Read the model definition and answer for the solid it produces. Units are mm, in the model's axes. Face numbers are marked on the shaded views. A direction names the side the tool comes from. Give positions to 0.01 mm unless a question says otherwise; leave off trailing zeros. Loops run counter-clockwise (first coordinate to the right, second up) from the corner with the lowest first, then second, coordinate; pieces in that order, holes last. Notation, with made-up numbers: (-11.75, 22) -> (6.25, 22) arc R12 ccw to (6.25, 33) -> close; hole circle Ø8 at (-15.5, 27). An arc over 180 degrees is marked (long way). Return JSON: item names as keys, results as strings. Group by question number.
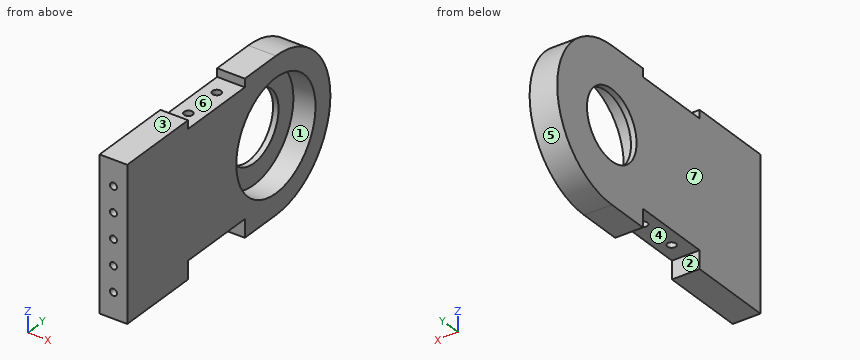
from build123d import *

# Parameters (mm, degrees)
BOSS_EXTRUDE1_DEPTH              = 20
SKETCH3_R                        = 40
CUT_EXTRUDE1_DEPTH               = 16
SKETCH4_R                        = 25
CUT_EXTRUDE2_DEPTH               = 11.1125
TAP_DRILL_FOR_M6X1_0_TAP2_D      = 5
TAP_DRILL_FOR_M6X1_0_TAP2_DEPTH  = 40
TAP_DRILL_FOR_M6X1_0_TAP2_TIP    = 1.502151548
SKETCH12_W                       = 6
SKETCH12_H                       = 57.3
SKETCH12_W_2                     = 13
CUT_EXTRUDE3_DEPTH               = 20
TAP_DRILL_FOR_M6_HELICOIL1_D     = 6.25
TAP_DRILL_FOR_M6_HELICOIL1_DEPTH = 20
TAP_DRILL_FOR_M6_HELICOIL1_TIP   = 1.877689434
TAP_DRILL_FOR_M6_HELICOIL2_D     = 6.25
TAP_DRILL_FOR_M6_HELICOIL2_DEPTH = 20
TAP_DRILL_FOR_M6_HELICOIL2_TIP   = 1.877689434


with BuildPart() as part:
    # Sketch2 → Boss-Extrude1 (new body)
    with BuildSketch(Plane(origin=(0, 0, 0), x_dir=(0, 0, -1), z_dir=(1, 0, 0))):
        with BuildLine():
            Line((55, -75), (55, 75))
            ThreePointArc((55, 75), (0, 20), (-55, 75))
            Line((-55, 75), (-55, -75))
            Line((-55, -75), (55, -75))
        make_face()
        with BuildLine():
            ThreePointArc((-55, 75), (0, 20), (55, 75))
            Line((55, 75), (-55, 75))
        make_face()
        with BuildLine():
            Line((-55, 75), (55, 75))
            ThreePointArc((55, 75), (0, 130), (-55, 75))
        make_face()
    extrude(amount=BOSS_EXTRUDE1_DEPTH)

    # Sketch3 → Cut-Extrude1 (cut)
    with BuildSketch(Plane(origin=(20, 0, 0), x_dir=(0, 0, -1), z_dir=(1, 0, 0))):
        with Locations((0, 75)):
            Circle(SKETCH3_R)
    extrude(amount=-CUT_EXTRUDE1_DEPTH, mode=Mode.SUBTRACT)

    # Sketch4 → Cut-Extrude2 (cut)
    with BuildSketch(Plane(origin=(4, 0, 0), x_dir=(0, 0, -1), z_dir=(1, 0, 0))):
        with Locations((0, 75)):
            Circle(SKETCH4_R)
    extrude(amount=-CUT_EXTRUDE2_DEPTH, mode=Mode.SUBTRACT)

    # Tap Drill for M6x1.0 Tap2
    with Locations(Plane(origin=(0, -75, 0), x_dir=(-1, 0, 0), z_dir=(0, -1, 0))):
        with Locations((-10, -36.666666667), (-10, -18.333333333), (-10, 0), (-10, 18.333333333), (-10, 36.666666667)):
            Hole(TAP_DRILL_FOR_M6X1_0_TAP2_D / 2, depth=TAP_DRILL_FOR_M6X1_0_TAP2_DEPTH)
            with Locations((0, 0, -(TAP_DRILL_FOR_M6X1_0_TAP2_DEPTH + TAP_DRILL_FOR_M6X1_0_TAP2_TIP / 2))):  # 118° drill point
                Cone(0, TAP_DRILL_FOR_M6X1_0_TAP2_D / 2, TAP_DRILL_FOR_M6X1_0_TAP2_TIP, mode=Mode.SUBTRACT)

    # Sketch12 → Cut-Extrude3 (cut)
    with BuildSketch(Plane(origin=(20, 0, 0), x_dir=(0, 0, -1), z_dir=(1, 0, 0))):
        with Locations((-52, 15)):
            Rectangle(SKETCH12_W, SKETCH12_H)
        with Locations((48.5, 15)):
            Rectangle(SKETCH12_W_2, SKETCH12_H)
    extrude(amount=-CUT_EXTRUDE3_DEPTH, mode=Mode.SUBTRACT)

    # Tap Drill for M6 Helicoil1
    with Locations(Plane(origin=(10, 29.325, 49), x_dir=(1, 0, 0), z_dir=(0, 0, 1))):
        with Locations((0, 0), (0, -28.65)):
            Hole(TAP_DRILL_FOR_M6_HELICOIL1_D / 2, depth=TAP_DRILL_FOR_M6_HELICOIL1_DEPTH)
            with Locations((0, 0, -(TAP_DRILL_FOR_M6_HELICOIL1_DEPTH + TAP_DRILL_FOR_M6_HELICOIL1_TIP / 2))):  # 118° drill point
                Cone(0, TAP_DRILL_FOR_M6_HELICOIL1_D / 2, TAP_DRILL_FOR_M6_HELICOIL1_TIP, mode=Mode.SUBTRACT)

    # Tap Drill for M6 Helicoil2
    with Locations(Plane(origin=(0, 0, -42), x_dir=(-1, 0, 0), z_dir=(0, 0, -1))):
        with Locations((-10, 29.325), (-10, 0.675)):
            Hole(TAP_DRILL_FOR_M6_HELICOIL2_D / 2, depth=TAP_DRILL_FOR_M6_HELICOIL2_DEPTH)
            with Locations((0, 0, -(TAP_DRILL_FOR_M6_HELICOIL2_DEPTH + TAP_DRILL_FOR_M6_HELICOIL2_TIP / 2))):  # 118° drill point
                Cone(0, TAP_DRILL_FOR_M6_HELICOIL2_D / 2, TAP_DRILL_FOR_M6_HELICOIL2_TIP, mode=Mode.SUBTRACT)


solid = part.part
1. Section D-D on z = -29 is taken. Determine the outline of the cut face in (x, y) (3 decimals).
2. Determine the mould class of the marked faces 4, 5, 6 and 7 for opening direction Y: pulls with the +Y half, pulls with the -Y half, needs draft (parallel to the pull), parting line crosses it, or undercut.
3. Section B-B on y = 62 is taken. Determine the outline of the cut face in (x, z), then the cut area to 3 significant figures.
4. Flat-ended cylindrical pins translate along their axes: pin 1 Ø4 at (x, z) = (12, -50.5) entering from +Y; pin 2 Ø1.5 at (x, y) = (5.5, -2.5) entering from -Z; pin 3 Ø10 at (x, y) = (10, 0.675) entering from +Z. Find the tip coordinate at first contact, or state that the pin passes through.
5. Section A-A on x = 17 is taken. Determine the outline of the cut face in (y, z), then the cut area to 3 significant figures.
6. Section C-C on z = -9.5 is taken. Determine the outline of the cut face in (x, y).
7. Which of the six approach directions +Z, -Z, +X, -X, +Y, -Y give full straight-line access (tool end or side, diameter ignored) to the marked faces 1, 2 and 3?
8. Straight lines are drawn through the part: line 1 (Z direction, x = 10, y = -45); line 2 (Y direction, x = 10, z = 43.75); line 3 (Y direction, x = 9.75, z = 31.5). For each, find the intervals that lie inside material, in ascending order. Write a range as from..to.
Completed:
{
 "1": {"outline": "(0, -75) -> (20, -75) -> (20, 47.45) -> (4, 47.45) -> (4, 102.55) -> (20, 102.55) -> (20, 121.733) -> (0, 121.733) -> close; hole circle Ø6.25 at (10, 0.675); hole circle Ø6.25 at (10, 29.325)"},
 "2": {"face 4": "undercut", "face 5": "pulls with the +Y half", "face 6": "undercut", "face 7": "needs draft"},
 "3": {"outline": "(0, -55) -> (20, -55) -> (20, -37.83) -> (4, -37.83) -> (4, -21.35) -> (0, -21.35) -> close; (0, 21.35) -> (4, 21.35) -> (4, 37.83) -> (20, 37.83) -> (20, 55) -> (0, 55) -> close", "area": "819 mm²"},
 "4": {"pin 1": "stops at y = 100.94", "pin 2": "stops at z = -42", "pin 3": "stops at z = 49"},
 "5": {"outline": "(-75, -55) -> (-13.65, -55) -> (-13.65, -42) -> (43.65, -42) -> (43.65, -55) -> (75, -55) arc R55 ccw to (75, 55) -> (43.65, 55) -> (43.65, 49) -> (-13.65, 49) -> (-13.65, 55) -> (-75, 55) -> close; hole circle Ø80 at (75, 0)", "area": "15,100 mm²"},
 "6": {"outline": "(0, -75) -> (20, -75) -> (20, 36.14) -> (4, 36.14) -> (4, 51.88) -> (0, 51.88) -> close; (0, 98.12) -> (4, 98.12) -> (4, 113.86) -> (20, 113.86) -> (20, 129.17) -> (0, 129.17) -> close"},
 "7": {"face 1": "+X", "face 2": "-Z, +X, -X", "face 3": "+Z, +X, -X, +Y, -Y"},
 "8": {"line 1": "z = -55..-39.17, -34.17..-20.83, -15.83..-2.5, 2.5..15.83, 20.83..34.17, 39.17..55", "line 2": "y = -75..-2.45, 3.8..26.2, 32.45..108.33", "line 3": "y = -75..-2.44, 3.79..26.21, 32.44..50.35, 99.65..120.09"}
}
